Drawing for the job (mm, zero at the part's lowest x, y, z). A direction names the side the tool comes from. Coordinates: 2 decimals unless noted, no trailing zeros. Write each loop counter-clockwise with the first axis right and the second up, starting at its lowest first coordinate (ties: lowest second). Pieces come first, ordered by that corner, then holes. Notation, with made-up numbers: M 72,38 L 131,38 A20 ccw 131,50 Z; hole C 62.25,28.25 d8. An arc over 180 degrees is marked long. Use a Markdown table: item, result. Add a question column.
Q1. Mould opens along Z. For the marked faces 3 and 4 say: released by +Z, released by -Z, zero draft, split by the parting line, or undercut.
Q2. Slice it at D-D on z = 11.5. Write the cut outline in (x, y) (1 decimal), then the cut area to 3 significant figures.
Q3. Slice it at C-C on x = 9. Write the cut outline in (y, z) (1 decimal), then the cut area to 3 significant figures.
Q4. Tool access for the marked faces 1 and 2: list every direction of +Z, -Z, +X, -X, +Y, -Y with a clear straight run to the whole face (end or side of a thin tool).
Q5. Wall check: L1, parallel to Z at x = 9.25, y = 8.25 (1 decimal); L2, parallel to X at y = 7.75, z = 6.5 (1 decimal); L3, parallel to Z at x = 2.25, y = 8.75 (1 decimal). Give the ranges that are in metal, low to high. Write a range as from..to.
Q6. Pin check, flat tips, straight feed: pin 1 Ø6 at (y, z) = (4.5, 3) entering from -X; pin 2 Ø1.6 at (y, z) = (1, 2) entering from -X; pin 3 Ø1.5 at (y, z) = (5, 3.5) entering from +X (1 decimal); pin 4 Ø1 at (x, y) = (8.5, 2) entering from +Z. Stop position of each tip, or through.
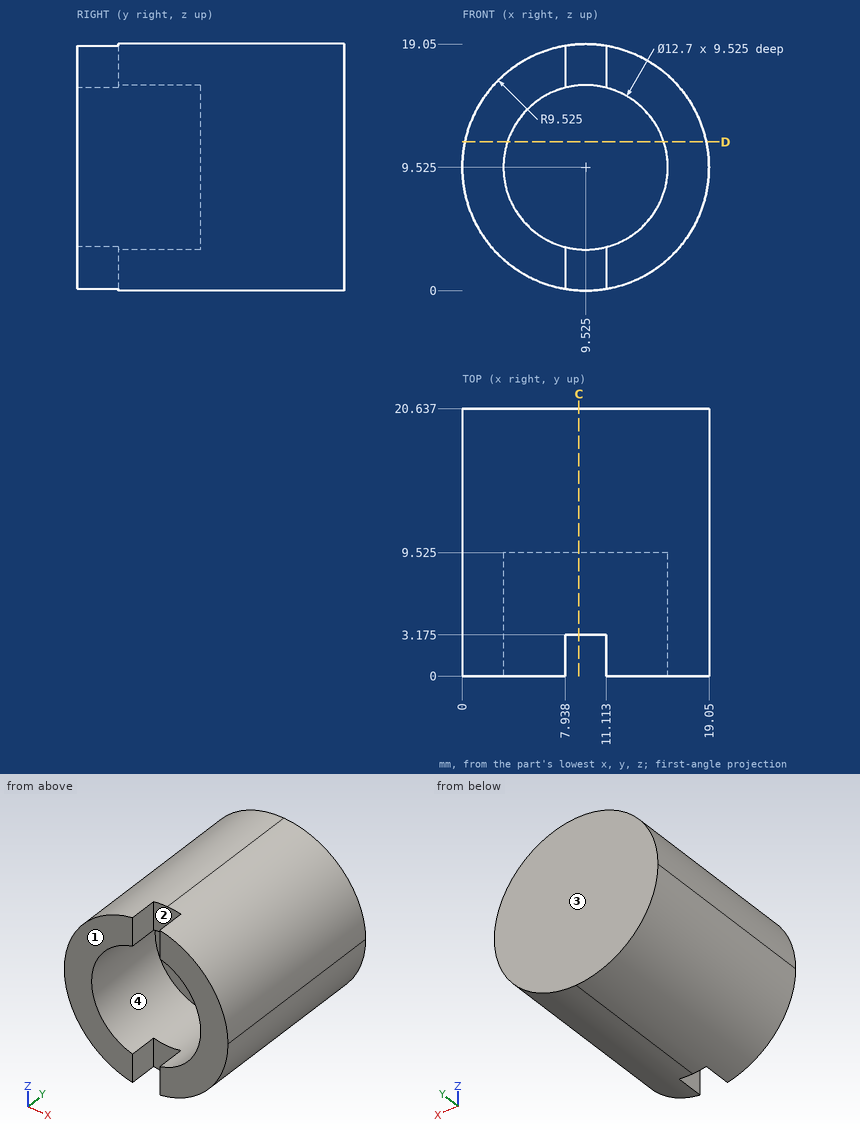
Recorded:
| question | item | result |
|---|---|---|
| 1 | face 3 | zero draft |
| 1 | face 4 | undercut |
| 2 | outline | M 0.2,0 L 3.5,0 L 3.5,9.5 L 15.6,9.5 L 15.6,0 L 18.8,0 L 18.8,20.6 L 0.2,20.6 Z |
| 2 | area | 270 mm² |
| 3 | outline | M 3.2,0 L 20.6,0 L 20.6,19 L 3.2,19 L 3.2,15.9 L 9.5,15.9 L 9.5,3.2 L 3.2,3.2 Z |
| 3 | area | 252 mm² |
| 4 | face 1 | +Z, -Z, +X, -X, -Y |
| 4 | face 2 | +Z, -Z, -Y |
| 5 | L1 | 0..3.2, 15.9..19 |
| 5 | L2 | 0.5..3.9, 15.1..18.6 |
| 5 | L3 | 3.4..15.7 |
| 6 | pin 1 | x = 0.68 |
| 6 | pin 2 | x = 2.78 |
| 6 | pin 3 | x = 17.5 |
| 6 | pin 4 | through |
